Check sheet for the modelled part. Datum: model origin and axes. Units: mm. Face numbers are marked on the shaded views. A direction names the side the tool comes from. Round coordinates to 2 decimals unless told otherwise and drop trailing zeros. Loops run counter-clockwise (first coordinate to the right, second up) from the corner with the lowest first, then second, coordinate; pieces in that order, holes last. Notation, with made-up numbers: (-23, 26) - (-3, 26) arc R18 ccw to (-3, 38) - close; hole circle Ø9 at (-27, -32). An arc over 180 degrees is marked (long way). Put each result on its own line as item: value.
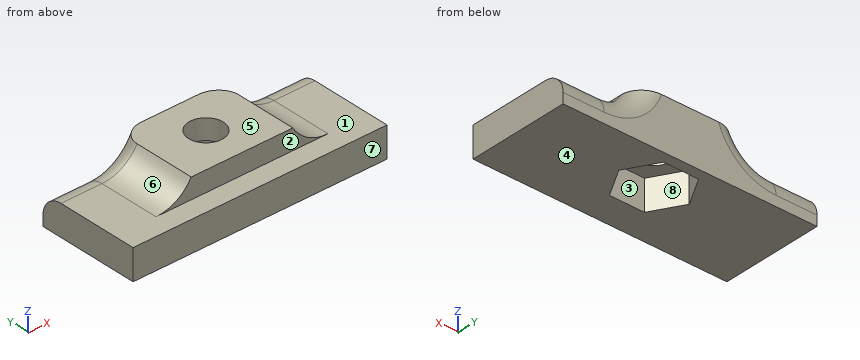
```python
from build123d import *

# Parameters (mm, degrees)
SKETCH2_W           = 25
SKETCH2_H           = 10
BOSS_EXTRUDE1_DEPTH = 3
SKETCH5_W           = 10
SKETCH5_H           = 8
BOSS_EXTRUDE3_DEPTH = 2
FILLET2_R           = 4
SKETCH8_R           = 1.7
CUT_EXTRUDE3_DEPTH  = 17.770509831
CUT_EXTRUDE4_DEPTH  = 3
FILLET3_R           = 2


with BuildPart() as part:
    # Sketch2 → Boss-Extrude1 (new body)
    with BuildSketch(Plane.XY):
        with Locations((0, 5)):
            Rectangle(SKETCH2_W, SKETCH2_H)
    extrude(amount=BOSS_EXTRUDE1_DEPTH)

    # Sketch5 → Boss-Extrude3 (add)
    with BuildSketch(Plane.XY.offset(3)):
        with Locations((0, 6)):
            Rectangle(SKETCH5_W, SKETCH5_H)
    extrude(amount=BOSS_EXTRUDE3_DEPTH)

    # Fillet2
    # the kernel refuses this fillet: 4 mm, written as the material it adds along each edge
    with BuildSketch(Plane(origin=(5, 10, 3), x_dir=(1, 0, 0), z_dir=(0, -1, 0)), Plane(origin=(-5, 2, 3), x_dir=(-1, 0, 0), z_dir=(0, 1, 0))) as fillet2_piece_1:
        with BuildLine():
            CenterArc((3.464101615, 4), FILLET2_R, 210, 60)
            Line((0, 2), (-0.069282032, 1.96))
            ThreePointArc((-0.069282032, 1.96), (-0.08, 1), (-0.08, 0))
            Line((-0.08, 0), (0, -0.08))
            Line((0, -0.08), (3.464101615, -0.08))
            Line((3.464101615, -0.08), (3.464101615, 0))
        make_face()
    extrude(amount=8)

    # Sketch8 → Cut-Extrude3 (cut, through all)
    with BuildSketch(Plane(origin=(0, 0, 0), x_dir=(-1, 0, 0), z_dir=(0, 0, -1))):
        with Locations((0, 6)):
            Circle(SKETCH8_R)
    extrude(amount=-CUT_EXTRUDE3_DEPTH, mode=Mode.SUBTRACT)

    # Sketch9 → Cut-Extrude4 (cut)
    with BuildSketch(Plane(origin=(0, 0, 0), x_dir=(-1, 0, 0), z_dir=(0, 0, -1))):
        Polygon((3.464101615, 6), (1.732050808, 9), (-1.732050808, 9), (-3.464101615, 6), (-1.732050808, 3), (1.732050808, 3), align=None)
    extrude(amount=-CUT_EXTRUDE4_DEPTH, mode=Mode.SUBTRACT)

    # Fillet3
    fillet3_edges = [part.edges().sort_by_distance(p)[0] for p in [
        (-10.482050808, 10, 3),
        (6.464101615, 10, 3.535898385),
        (-6.464101615, 10, 3.535898385),
        (10.482050808, 10, 3),
    ]]
    fillet(fillet3_edges, radius=FILLET3_R)


solid = part.part
```
Item 1: Thickness scan on line 1 (Y direction, x = 0, z = 4); line 2 (Z direction, x = 10.5, y = 2.5); line 3 (X direction, y = 7.75, z = 0.55). Record the ranges inside material, lowest first. Write a range as from..to.
Filled sheet:
line 1: 2..4.3, 7.7..10
line 2: 0..3
line 3: -12.5..-2.45, 2.45..12.5
Item 2: Section check A-A on x = 0. Enter the section's corners in (y, z).
Filled sheet:
outline: (0, 0) - (3, 0) - (3, 3) - (4.3, 3) - (4.3, 5) - (2, 5) - (2, 3) - (0, 3) - close; (7.7, 3) - (9, 3) - (9, 0) - (10, 0) - (10, 5) - (7.7, 5) - close
Item 3: Release check for a two-part mould opening along Y. For the marked faces 6, 7 and 8 record: +Y half, -Y half, draft (parallel to the pull), parting line (faces both ways), or undercut.
Filled sheet:
face 6: draft
face 7: -Y half
face 8: undercut
Item 4: Section check C-C on y = 3.25. Enter the section's corners in (x, z), then the cut area to 3 significant figures.
Filled sheet:
outline: (-12.5, 0) - (-1.88, 0) - (-1.88, 3) - (1.88, 3) - (1.88, 0) - (12.5, 0) - (12.5, 3) - (8.46, 3) arc R4 cw to (5, 5) - (-5, 5) arc R4 cw to (-8.46, 3) - (-12.5, 3) - close
area: 87.8 mm²
Item 5: Tool access check on the marked faces 1, 2, 3, 4 and 5. Record the directions out of +Z, -Z, +X, -X, +Y, -Y that give a thin tool (end or side, any length) a straight path to the whole face; none if there is none.
Filled sheet:
face 1: +Z, -Y
face 2: +Z, +X, -X, -Y
face 3: -Z
face 4: -Z, +X, -X, +Y, -Y
face 5: +Z, +X, -X, +Y, -Y
Item 6: Go/stop test with flat-tipped pins: pin 1 (4 mm diameter, centred on x = 10, y = 1, fed in from +Z); pin 2 (3 mm diameter, centred on x = 0.5, y = 6.5, fed in from -Z); pin 3 (2 mm diameter, centred on x = -3.5, z = 4.5, fed in from -Y). Record where each tip stops, or that it passes through.
Filled sheet:
pin 1: z = 3
pin 2: z = 3
pin 3: y = 2
Item 7: Section check B-B on y = 4.75. Enter the section's corners in (x, z).
Filled sheet:
outline: (-12.5, 0) - (-2.74, 0) - (-2.74, 3) - (-1.15, 3) - (-1.15, 5) - (-5, 5) arc R4 cw to (-8.46, 3) - (-12.5, 3) - close; (1.15, 3) - (2.74, 3) - (2.74, 0) - (12.5, 0) - (12.5, 3) - (8.46, 3) arc R4 cw to (5, 5) - (1.15, 5) - close
